```python
from build123d import *

# Parameters (mm, degrees)
SKETCH1_R           = 1.5
SKETCH1_R_2         = 1.25
BOSS_EXTRUDE1_DEPTH = 2.5
SKETCH2_R           = 4.375
SKETCH2_R_2         = 2.85
BOSS_EXTRUDE2_DEPTH = 2.5


with BuildPart() as part:
    # Sketch1 → Boss-Extrude1 (new body)
    with BuildSketch(Plane.XY):
        with BuildLine():
            Line((0.841414718, 4.928693668), (0, 5))
            ThreePointArc((0, 5), (-5, 0), (0, -5))
            Line((0, -5), (0.841414718, -4.928693668))
            Line((0.841414718, -4.928693668), (29.5, -2.5))
            ThreePointArc((29.5, -2.5), (32, 0), (29.5, 2.5))
            Line((29.5, 2.5), (0.841414718, 4.928693668))
        make_face()
        Circle(SKETCH1_R, mode=Mode.SUBTRACT)
        with Locations((15, 0)):
            Circle(SKETCH1_R_2, mode=Mode.SUBTRACT)
        with Locations((20, 0)):
            Circle(SKETCH1_R_2, mode=Mode.SUBTRACT)
        with Locations((25, 0)):
            Circle(SKETCH1_R_2, mode=Mode.SUBTRACT)
        with Locations((30, 0)):
            Circle(SKETCH1_R_2, mode=Mode.SUBTRACT)
    extrude(amount=BOSS_EXTRUDE1_DEPTH)

    # Sketch2 → Boss-Extrude2 (add)
    with BuildSketch(Plane(origin=(0, 0, 0), x_dir=(-1, 0, 0), z_dir=(0, 0, -1))):
        with Locations(Location((0, 0, 0), (0, 0, 180))):
            Circle(SKETCH2_R)
        Circle(SKETCH2_R_2, mode=Mode.SUBTRACT)
    extrude(amount=BOSS_EXTRUDE2_DEPTH)


solid = part.part
```
Source: CAD feature listing. Evaluate the final solid. Frame: model axes, mm. A direction names the side the tool comes from. Give positions to 0.01 mm unless a question says otherwise; leave off trailing zeros. Order: outer loops, then holes, each group sorted by start corner. A loop starts at its lowest first (then second) coordinate and runs counter-clockwise, first axis right, second up. Notation, with made-up numbers: (2.25, 47) -> (56.25, 47) arc R11 cw to (56.25, 61) -> close; hole circle Ø9 at (-32.75, 40.25). An arc over 180 degrees is marked (long way). Use a Markdown table: item, result.
Q1. Section A-A (y = 0). State how many separate pieces and enclosed holes the cut face has, and give its area (3 significant figures).
A:
| item | result |
|---|---|
| separate pieces | 6 |
| enclosed holes | 0 |
| area | 67.6 mm^2 |
Q2. Section D-D (y = 3.75). Return the cut outline in (x, z), and give its area (3 significant figures).
A:
| item | result |
|---|---|
| outline | (-3.31, 0) -> (-2.25, 0) -> (-2.25, -2.5) -> (2.25, -2.5) -> (2.25, 0) -> (14.75, 0) -> (14.75, 2.5) -> (-3.31, 2.5) -> close |
| area | 56.4 mm^2 |
Q3. Pull-direction query (X, two-part tool) for faces 1 (the face through (9, 0, 2.5)), 2 (the face through (32, 0, 1)), 3 (the face through (-5, 0, 1)), 4 (the face through (13.75, 0.05, 1.23)); classes: +X half, -X half, draft (parallel to the pull), parting line (faces both ways), or undercut.
A:
| item | result |
|---|---|
| face 1 | draft |
| face 2 | +X half |
| face 3 | -X half |
| face 4 | undercut |
Q4. Section C-C (x = 25). Return the cut outline in (y, z), and give its area (3 significant figures).
A:
| item | result |
|---|---|
| outline | (-2.88, 0) -> (-1.25, 0) -> (-1.25, 2.5) -> (-2.88, 2.5) -> close; (1.25, 0) -> (2.88, 0) -> (2.88, 2.5) -> (1.25, 2.5) -> close |
| area | 8.16 mm^2 |
Q5. Section B-B (z = 0.75). Return the cut outline in (x, y), and give its area (3 significant figures).
A:
| item | result |
|---|---|
| outline | (0, -5) -> (29.5, -2.5) arc R2.5 ccw to (29.5, 2.5) -> (0, 5) arc R5 ccw to start; hole circle Ø3 at (0, 0); hole circle Ø2.5 at (15, 0); hole circle Ø2.5 at (20, 0); hole circle Ø2.5 at (25, 0); hole circle Ø2.5 at (30, 0) |
| area | 244 mm^2 |
Q6. First-contact query: P1, Ø3, axis at x = 10.5, y = 2, coming from the -Z side; P2, Ø2, axis at x = 20, z = 0, coming from the -Y side; P3, Ø1, axis at y = 1.5, z = 1.5, coming from the +X side. Flat tips, straight axial feed; report the tip coordinate or a pass-through.
A:
| item | result |
|---|---|
| P1 | z = 0 |
| P2 | y = -3.39 |
| P3 | x = 31.79 |
Q7. Access query for faces 5 (the face through (1.2, -1.2, 0)), 6 (the face through (26.155, -0.479, 1.232)). Directions: +Z, -Z, +X, -X, +Y, -Y. A direction counts if a zero-diameter tool reaches every point of the face in a straight line with its end or side. Return the directions, or none.
A:
| item | result |
|---|---|
| face 5 | -Z |
| face 6 | +Z, -Z |
Q8. Material intervals for line 1 (Y direction, x = 0, z = -0.9) (3 decimals); line 2 (Y direction, x = 0, z = 1.9); line 3 (X direction, y = -1, z = 1), sorted ascending. Write a range as [from, to].
A:
| item | result |
|---|---|
| line 1 | [-4.375, -2.85], [2.85, 4.375] |
| line 2 | [-5, -1.5], [1.5, 5] |
| line 3 | [-4.9, -1.12], [1.12, 14.25], [15.75, 19.25], [20.75, 24.25], [25.75, 29.25], [30.75, 31.79] |
